The listing builds one solid part. Answer for the finished solid, in the listing's coordinates (mm). Face numbers are marked on the shaded views. A direction names the side the tool comes from. Round coordinates to 2 decimals unless told otherwise and drop trailing zeros. Write each loop counter-clockwise with the first axis right and the second up, starting at its lowest first coordinate (ties: lowest second). Pieces come first, ordered by that corner, then holes. Notation, with made-up numbers: (73, -22) -> (94, -22) arc R18 cw to (94, 4) -> close; hole circle Ø1 at (86, -12.75). An arc over 180 degrees is marked (long way). Write each question's results on one line, items separated by ' | '. Start each with the question number.
Autodesk Inventor part; units mm, degrees
ref_plane "YZ Plane" through (0, 0, 0) normal (1, 0, 0) x (0, 1, 0)
ref_plane "XZ Plane" through (0, 0, 0) normal (0, 1, 0) x (-1, 0, 0)
ref_plane "XY Plane" through (0, 0, 0) normal (0, 0, 1) x (1, 0, 0)
sketch "Эскиз1" plane through (0, 0, 0) normal (0, 0, 1) x (1, 0, 0)
  arc A0 (9.8, 10) -> (7.8, 12) centre (7.8, 10) ccw
  line L0 (2, 12) -> (7.8, 12)
  arc A1 (2, 12) -> (0, 10) centre (2, 10) ccw
  line L1 (0, 0) -> (0, 10)
  line L2 (9.8, 0) -> (0, 0)
  line L3 (9.8, 0) -> (9.8, 10)
  line L4 (2.05, 7.1454) -> (4.9, 8.7909)
  line L5 (4.9, 8.7909) -> (7.75, 7.1454)
  line L6 (7.75, 7.1454) -> (7.75, 3.8546)
  line L7 (7.75, 3.8546) -> (4.9, 2.2091)
  line L8 (4.9, 2.2091) -> (2.05, 3.8546)
  line L9 (2.05, 3.8546) -> (2.05, 7.1454)
  circle A2 centre (4.9, 5.5) radius 1.7
  circle A3 centre (4.9, 5.5) radius 1.5
  dimension "d0" = 3
extrude "Выдавливание1" add sketch "Эскиз1" along normal blind 4.2 contours L3 L2 L1 A1 L0 A0 | L4 L5 L6 L7 L8 L9 | A2 | A3
sketch "Эскиз2" plane through (0, 0, 4.2) normal (0, 0, 1) x (1, 0, 0)
  line L0 (0, 10) -> (0, 0)
  line L1 (9.8, 0) -> (9.8, 10)
  line L2 (0, 7.2) -> (9.8, 7.2)
  line L3 (9.8, 7.2) -> (9.8, 1)
  line L4 (9.8, 1) -> (0, 1)
  line L5 (0, 1) -> (0, 7.2)
  line L6 (0, 0) -> (9.8, 0)
  dimension "d3" = 1
  dimension "d4" = 6.2
extrude "Выдавливание2" cut sketch "Эскиз2" against normal blind 1 contours L2 L1 L4 L0
sketch "Эскиз3" plane through (2, 12, 0) normal (0, 1, 0) x (1, 0, 0)
  line L0 (5.8, 0) -> (5.8, -4.2)
  line L1 (0, 0) -> (5.8, 0)
  line L2 (5.8, 0) -> (0, 0)
  line L3 (2.9, 0) -> (2.9, -1.6661)
  line L4 (3.9, 0) -> (1.9, 0)
  line L5 (1.9, 0) -> (1.9, -1)
  line L6 (1.9, -1) -> (3.9, -1)
  line L7 (3.9, -1) -> (3.9, 0)
  line L8 (3.9, 0) -> (1.9, 0)
  line L9 (1.9, 0) -> (1.9, 2)
  line L10 (1.9, 2) -> (3.9, 2)
  line L11 (3.9, 2) -> (3.9, 0)
  point P0 (-2, 0)
  dimension "d7" = 2
  dimension "d8" = 1
  dimension "d9" = 2
extrude "Выдавливание3" add sketch "Эскиз3" against normal up to surface (12 mm away) contours L9 L10 L11 L1
properties part number "натяжитель ремня"
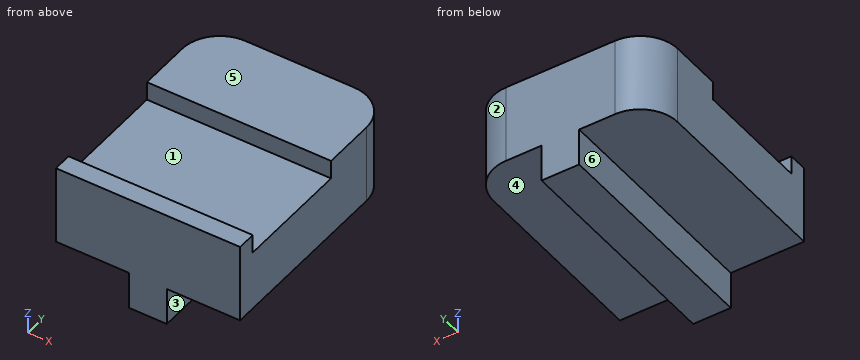
Q1. Determine the mould class of the marked faces 1, 2 and 3 for opening direction Y: pulls with the +Y half, pulls with the -Y half, needs draft (parallel to the pull), parting line crosses it, or undercut.
Q2. The part is cut by section D-D, the plane z = -1. Write down the section's boundary in (x, y).
Q3. Find the intervals of material crossed by line 1 (Y direction, x = 2.5, z = 3.5); line 2 (X direction, y = 10.5, z = -0.75); line 3 (Z direction, x = 6.75, y = 6.5), in increasing order.
Q4. For the marked faces 4, 5 and 6, determine the directions among +Z, -Z, +X, -X, +Y, -Y from which every point of the face is accessible in a straight line to the end or side of a thin tool.
Q5. The part is cut by section B-B, the plane y = 9.5. Write down the section's boundary in (x, z).
Q6. The part is cut by section A-A, the plane z = 3.5. Write down the section's boundary in (x, y).
Q7. Each of these flat-tipped pins is pushed along its axis until it touches: pin 1 (1.6 mm diameter, centred on y = 4.5, z = -1, fed in from +X); pin 2 (1.2 mm diameter, centred on x = 1.5, y = 7, fed in from -Z); pin 3 (1 mm diameter, centred on y = 8, z = -1, fed in from -X). Where does it stop, or does it pass through?
Q8. The part is cut by section C-C, the plane x = 6.25. Write down the section's boundary in (y, z), then the cut area to 3 significant figures.
Answers follow:
1) face 1: undercut | face 2: pulls with the +Y half | face 3: needs draft
2) outline: (3.9, 0) -> (5.9, 0) -> (5.9, 12) -> (3.9, 12) -> close
3) line 1: 0 to 1, 7.2 to 12 | line 2: 3.9 to 5.9 | line 3: 0 to 3.2
4) face 4: -Z, +X, +Y, -Y | face 5: +Z, +X, -X, +Y, -Y | face 6: -Z, -X, +Y, -Y
5) outline: (0, 0) -> (3.9, 0) -> (3.9, -2) -> (5.9, -2) -> (5.9, 0) -> (9.8, 0) -> (9.8, 4.2) -> (0, 4.2) -> close
6) outline: (0, 0) -> (9.8, 0) -> (9.8, 1) -> (0, 1) -> close; (0, 7.2) -> (9.8, 7.2) -> (9.8, 10) arc R2 ccw to (7.8, 12) -> (2, 12) arc R2 ccw to (0, 10) -> close
7) pin 1: x = 5.9 | pin 2: z = 0 | pin 3: x = 3.9
8) outline: (0, 0) -> (12, 0) -> (12, 4.2) -> (7.2, 4.2) -> (7.2, 3.2) -> (1, 3.2) -> (1, 4.2) -> (0, 4.2) -> close | area: 44.2 mm^2
